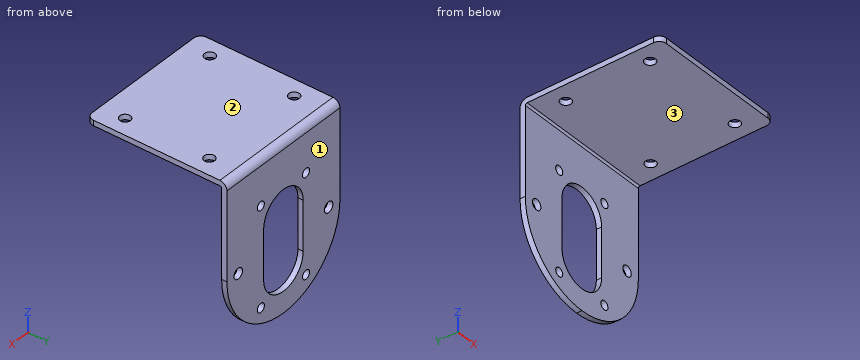
Autodesk Inventor part; units mm, degrees
ref_plane "YZ Plane" through (0, 0, 0) normal (1, 0, 0) x (0, 1, 0)
ref_plane "XZ Plane" through (0, 0, 0) normal (0, 1, 0) x (-1, 0, 0)
ref_plane "XY Plane" through (0, 0, 0) normal (0, 0, 1) x (1, 0, 0)
sketch "Sketch1" plane through (0, 0, 0) normal (1, 0, 0) x (0, 1, 0)
  line L0 (0, 0) -> (38, 0)
  line L1 (40, -2) -> (40, -47)
  arc A0 (40, -2) -> (38, 0) centre (38, -2) ccw
  line L2 (38.5, -47) -> (38.5, -2)
  arc A1 (38.5, -2) -> (38, -1.5) centre (38, -2) ccw
  line L3 (38, -1.5) -> (0, -1.5)
  line L4 (40, -47) -> (38.5, -47)
  line L5 (0, 0) -> (0, -1.5)
  point P0 (40, 0)
  dimension "d0" = 47
  dimension "d1" = 40
  dimension "d2" = 2
  dimension "d3" = 1.5
extrude "Extrusion1" add sketch "Sketch1" along normal mid plane 40
fillet "Fillet1" radius 20 2 edges at (20, 39.25, -47) (-20, 39.25, -47)
fillet "Fillet2" radius 2 2 edges at (-20, 0, -0.75) (20, 0, -0.75)
sketch "Sketch2" plane through (-20, 38, 0) normal (0, 0, 1) x (1, 0, 0)
  circle A0 centre (5, -7) radius 1.5
  circle A1 centre (5, -31) radius 1.5
  circle A2 centre (35, -31) radius 1.5
  circle A3 centre (35, -7) radius 1.5
  point P0 (20, -38)
extrude "Extrusion2" cut sketch "Sketch2" against normal through all
sketch "Sketch3" plane through (-20, 40, -2) normal (0, 1, 0) x (1, 0, 0)
  arc A0 (13, 18) -> (27, 18) centre (20, 18) ccw
  arc A1 (27, 32) -> (13, 32) centre (20, 32) ccw
  line L0 (13, 18) -> (13, 32)
  line L1 (27, 18) -> (27, 32)
  arc A2 (40, 25) -> (0, 25) centre (20, 25) ccw
  circle A3 centre (36, 25) radius 1.5
  circle A4 centre (4, 25) radius 1.5
  circle A5 centre (28, 11) radius 1.25
  circle A6 centre (12, 11) radius 1.25
  line L2 (40, 0) -> (40, 25)
  line L3 (40, 25) -> (0, 25)
  circle A7 centre (28, 39) radius 1.25
  circle A8 centre (12, 39) radius 1.25
  point P0 (20, -2)
  dimension "d10" = 14
  dimension "d11" = 14
  dimension "d12" = 28
  dimension "d13" = 7
  dimension "d14" = 3
  dimension "d15" = 3
  dimension "d16" = 32
  dimension "d17" = 16
  dimension "d18" = 2.5
  dimension "d19" = 2.5
  dimension "d20" = 16
  dimension "d21" = 8
extrude "Extrusion3" cut sketch "Sketch3" against normal through all contours L0 L3 L1 A0 | L0 A1 L1 L3 | L3 A4 | A4 L3 | L3 A3 | A3 L3 | A5 | A6 | A7 | A8
equation "\"d17\" = 0.5 * d16"
equation "\"d21\" = 0.5 * d20"
properties part number "MotorMount"
Work out the finished part from the listing and answer in its coordinate system (mm). Face numbers are marked on the shaded views. Give positions to 0.01 mm unless a question says otherwise; leave off trailing zeros. Loops run counter-clockwise (first coordinate to the right, second up) from the corner with the lowest first, then second, coordinate; pieces in that order, holes last. Notation, with made-up numbers: M -34,62 L -30,62 A9 cw -30,69 Z; hole C 20.5,-36.5 d2. An arc over 180 degrees is marked long. One line per item, written item: value. Start each with the question number.
1. Find section A-A (y = 7). Give the vertices of the cut face in (x, z).
2. Find section C-C (z = -15). Give the vertices of the cut face in (x, y).
3. Each of these flat-tipped pins is pushed along its axis until it touches: P1, Ø2.5, axis at x = 16, z = -27, coming from the +Y side; P2, Ø10, axis at x = 13, z = -16.5, coming from the -Y side; P3, Ø6, axis at x = -11.5, y = 6.5, coming from the -Z side; P4, Ø3, axis at x = 8, z = -13, coming from the +Y side. Where does it stop, or does it pass through?
4. Find section B-B (x = -6). Give the vertices of the cut face in (y, z).
5. Find section D-D (x = 5). Give the vertices of the cut face in (y, z), and give its area (3 significant figures).
6. Find the intervals of material crossed by probe 1 along Y at (x, z) = (15, -0.6); probe 2 along Y at (x, z) = (-13, -21); probe 3 along Z at (x, y) = (-10.5, 20.5), in increasing order.
7. Determine the mould class of the marked faces 1, 2 and 3 for opening direction Z: released by +Z, released by -Z, zero draft, split by the parting line, or undercut.
Reported:
1. outline: M -20,-1.5 L -16.5,-1.5 L -16.5,0 L -20,0 Z; M -13.5,-1.5 L 13.5,-1.5 L 13.5,0 L -13.5,0 Z; M 16.5,-1.5 L 20,-1.5 L 20,0 L 16.5,0 Z
2. outline: M -20,38.5 L -4.9,38.5 L -4.9,40 L -20,40 Z; M 4.9,38.5 L 20,38.5 L 20,40 L 4.9,40 Z
3. P1: passes through
3. P2: stops at y = 38.5
3. P3: stops at z = -1.5
3. P4: stops at y = 40
4. outline: M 0,-1.5 L 38,-1.5 A0.5 cw 38.5,-2 L 38.5,-16.39 L 40,-16.39 L 40,-2 A2 ccw 38,0 L 0,0 Z; M 38.5,-46.08 L 40,-46.08 L 40,-37.61 L 38.5,-37.61 Z
5. outline: M 0,-1.5 L 38,-1.5 A0.5 cw 38.5,-2 L 38.5,-15.1 L 40,-15.1 L 40,-2 A2 ccw 38,0 L 0,0 Z; M 38.5,-46.37 L 40,-46.37 L 40,-38.9 L 38.5,-38.9 Z
5. area: 90.8 mm²
6. probe 1: y = 0 to 5.5, 8.5 to 29.5, 32.5 to 39.43
6. probe 2: y = 38.5 to 40
6. probe 3: z = -1.5 to 0
7. face 1: zero draft
7. face 2: released by +Z
7. face 3: released by -Z
